```python
from build123d import *

# Parameters (mm, degrees)
EXTRUDE_1_DEPTH = 20
SKETCH_3_R      = 1.5
EXTRUDE_2_DEPTH = 3


with BuildPart() as part:
    # Эскиз1 → Бобышка-Вытянуть1 (new body)
    with BuildSketch(Plane.XY):
        with BuildLine():
            Line((-0.706664701, 9.975), (-0.706664701, 12.975))
            ThreePointArc((-0.706664701, 12.975), (-12.994229489, 0), (-0.706664701, -12.975))
            Line((-0.706664701, -12.975), (-0.706664701, -9.975))
            ThreePointArc((-0.706664701, -9.975), (-10, 0), (-0.706664701, 9.975))
        make_face()
    extrude(amount=EXTRUDE_1_DEPTH)

    # Эскиз3 → Бобышка-Вытянуть2 (add)
    # profile 1 of 2: a face of its own
    with BuildSketch(Plane(origin=(-0.706664701, 0, 0), x_dir=(0, 0, -1), z_dir=(1, 0, 0))):
        Polygon((-10, 9.975), (-14.5, 9.975), (-14.5, 21.975), (-5.5, 21.975), (-5.5, 9.975), align=None)
        with Locations((-10, 17.475)):
            Circle(SKETCH_3_R, mode=Mode.SUBTRACT)
    # profile 2 of 2: a face of its own
    with BuildSketch(Plane(origin=(-0.706664701, 0, 0), x_dir=(0, 0, -1), z_dir=(1, 0, 0))):
        Polygon((-10, -9.975), (-14.5, -9.975), (-14.5, -21.975), (-5.5, -21.975), (-5.5, -9.975), align=None)
        with Locations((-10, -17.475)):
            Circle(SKETCH_3_R, mode=Mode.SUBTRACT)
    extrude(amount=-EXTRUDE_2_DEPTH)


solid = part.part
```
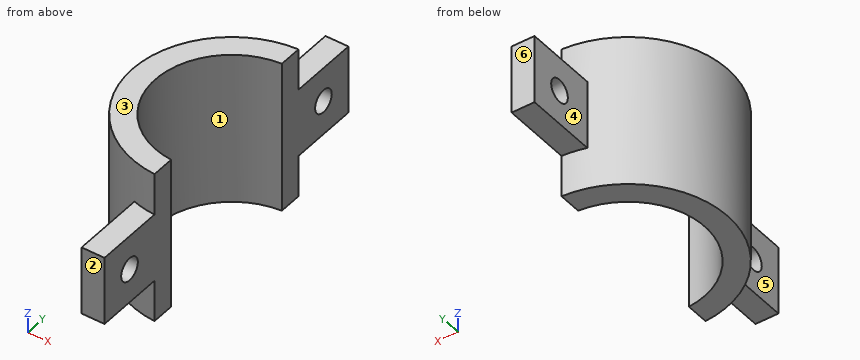
Here's how the part is built. I have some questions about the finished solid (model axes, mm). Face numbers are marked on the shaded views. A direction names the side the tool comes from. Coordinates: 2 decimals unless noted, no trailing zeros. Loops run counter-clockwise (first coordinate to the right, second up) from the corner with the lowest first, then second, coordinate; pieces in that order, holes last. Notation, with made-up numbers: (-25.75, 36) - (26.25, 36) arc R26 ccw to (26.25, 75) - close; hole circle Ø2 at (-33, 29.5). An arc over 180 degrees is marked (long way). Answer as CSV lines item,"result".
Q1. We'd pull the mould along Y, two halves only. Please class the marked faces 1, 2 and 3: pulls with the +Y half, pulls with the -Y half, needs draft (parallel to the pull), parting line crosses it, or undercut.
Response:
face 1,"undercut"
face 2,"pulls with the -Y half"
face 3,"needs draft"
Q2. If we section it at A-A, the plane z = 10: Write out the boundary of the cut face in (x, y) (3 decimals).
Response:
outline,"(-3.707, -21.975) - (-0.707, -21.975) - (-0.707, -18.975) - (-3.707, -18.975) - close; (-3.707, -15.975) - (-0.707, -15.975) - (-0.707, -9.975) arc R10 cw to (-0.707, 9.975) - (-0.707, 15.975) - (-3.707, 15.975) - (-3.707, 12.454) arc R12.994 ccw to (-3.707, -12.454) - close; (-3.707, 18.975) - (-0.707, 18.975) - (-0.707, 21.975) - (-3.707, 21.975) - close"
Q3. For pin 1 (4.5 mm diameter, centred on y = 17.5, z = 9, fed in from -X); pin 2 (0.9 mm diameter, centred on x = -2, y = -18, fed in from +Z); pin 3 (2.5 mm diameter, centred on x = -2, y = -15, fed in from -Z), each with a flat end and sliding along its axis, tell me the tip position at first contact or that it passes through.
Response:
pin 1,"x = -3.71"
pin 2,"z = 14.5"
pin 3,"z = 5.5"
Q4. If we section it at B-B, the plane x = -2.75: Write out the boundary of the cut face in (y, z) (3 decimals).
Response:
outline,"(-21.975, 5.5) - (-12.7, 5.5) - (-12.7, 0) - (-9.614, 0) - (-9.614, 20) - (-12.7, 20) - (-12.7, 14.5) - (-21.975, 14.5) - close; (9.614, 0) - (12.7, 0) - (12.7, 5.5) - (21.975, 5.5) - (21.975, 14.5) - (12.7, 14.5) - (12.7, 20) - (9.614, 20) - close; hole circle Ø3 at (-17.475, 10); hole circle Ø3 at (17.475, 10)"
Q5. If we section it at C-C, the plane x = -6.25: Write out the boundary of the cut face in (y, z).
Response:
outline,"(-11.39, 0) - (-7.81, 0) - (-7.81, 20) - (-11.39, 20) - close; (7.81, 0) - (11.39, 0) - (11.39, 20) - (7.81, 20) - close"
Q6. If I drill on L1, parallel to Y at x = -2.7, z = 10 (3 decimals); L2, parallel to Y at x = -1.9, z = 10 (3 decimals); L3, parallel to Z at x = -3.5, y = 14, over which ranges is the centre line in solid material (lowest first)? Write a range as [from, to].
Response:
L1,"[-21.975, -18.975], [-15.975, -9.629], [9.629, 15.975], [18.975, 21.975]"
L2,"[-21.975, -18.975], [-15.975, -9.818], [9.818, 15.975], [18.975, 21.975]"
L3,"[5.5, 14.5]"
Q7. If we section it at D-D, the plane y = 0: Write out the boundary of the cut face in (x, z).
Response:
outline,"(-12.99, 0) - (-10, 0) - (-10, 20) - (-12.99, 20) - close"
Q8. For the marked faces 4, 5 and 6, which set-ups out of +Z, -Z, +X, -X, +Y, -Y let a thin tool reach every point of the face, with its end or its side?
Response:
face 4,"+Z, -Z, -X, +Y"
face 5,"+Z, -Z, -X, -Y"
face 6,"+Z, -Z, +X, -X, +Y"
